Source: CAD feature listing. Evaluate the final solid. Frame: model axes, mm. A direction names the side the tool comes from. Give positions to 0.01 mm unless a question says otherwise; leave off trailing zeros. Loops run counter-clockwise (first coordinate to the right, second up) from the corner with the lowest first, then second, coordinate; pieces in that order, holes last. Notation, with made-up numbers: (-20, 81) - (13, 81) arc R23 cw to (13, 112) - close; hole circle Ø7 at (23.25, 8). An arc over 180 degrees is marked (long way). Put each result on its own line as item: value.
```python
from build123d import *

# Parameters (mm, degrees)
SKETCH1_W            = 152.4
SKETCH1_H            = 254
BOSS_EXTRUDE1_DEPTH  = 12.7
SKETCH2_W            = 38.1
SKETCH2_H            = 19.05
CUT_EXTRUDE1_DEPTH   = 149.649688866
FILLET1_R            = 3.302
FILLET1_OF_MIRROR1_R = 3.302
FILLET2_R            = 3.302


with BuildPart() as part:
    # Sketch1 → Boss-Extrude1 (new body)
    with BuildSketch(Plane(origin=(0, 0, 0), x_dir=(1, 0, 0), z_dir=(0, 1, 0))):
        Rectangle(SKETCH1_W, SKETCH1_H)
    extrude(amount=BOSS_EXTRUDE1_DEPTH)

    # Sketch2 → Cut-Extrude1 (cut, through all)
    with BuildSketch(Plane(origin=(0, 12.7, 0), x_dir=(1, 0, 0), z_dir=(0, 1, 0))):
        with Locations((57.15, -66.675)):
            Rectangle(SKETCH2_W, SKETCH2_H)
    cut_extrude1 = extrude(amount=-CUT_EXTRUDE1_DEPTH, mode=Mode.SUBTRACT)

    # Fillet1
    fillet1_edges = [part.edges().sort_by_distance(p)[0] for p in [
        (38.1, 6.35, 76.2),
        (38.1, 6.35, 57.15),
    ]]
    fillet(fillet1_edges, radius=FILLET1_R)

    # Mirror1: Cut-Extrude1 across plane
    add(cut_extrude1.mirror(Plane(origin=(0, 0, 0), x_dir=(0, 0, 1), z_dir=(1, 0, 0))), mode=Mode.SUBTRACT)

    # Fillet1 of Mirror1
    fillet1_of_mirror1_edges = [part.edges().sort_by_distance(p)[0] for p in [
        (-38.1, 6.35, 76.2),
        (-38.1, 6.35, 57.15),
    ]]
    fillet(fillet1_of_mirror1_edges, radius=FILLET1_OF_MIRROR1_R)

    # Fillet2
    fillet2_edges = [part.edges().sort_by_distance(p)[0] for p in [
        (76.2, 6.35, 57.15),
        (76.2, 6.35, 76.2),
        (-76.2, 6.35, 76.2),
        (-76.2, 6.35, 57.15),
        (76.2, 6.35, 127),
        (-76.2, 6.35, 127),
        (-76.2, 6.35, -127),
        (76.2, 6.35, -127),
    ]]
    fillet(fillet2_edges, radius=FILLET2_R)


solid = part.part
```
1) Section query A-A, the plane x = 58. Output: boundary loops of the cut face in (y, z), plus the area to 3 significant figures.
Check result:
outline: (0, -127) - (12.7, -127) - (12.7, 57.15) - (0, 57.15) - close; (0, 76.2) - (12.7, 76.2) - (12.7, 127) - (0, 127) - close
area: 2,980 mm²
2) Pin query (flat end, axial travel): P1, Ø6, axis at y = 8.5, z = 68.5, coming from the +X side. Return the tip coordinate at first contact, or that it passes through.
Check result:
P1: x = 38.1
3) Section query B-B, the plane y = 5.75. Output: boundary loops of the cut face in (x, z), plus the area to 3 significant figures.
Check result:
outline: (-76.2, -123.7) arc R3.3 ccw to (-72.9, -127) - (72.9, -127) arc R3.3 ccw to (76.2, -123.7) - (76.2, 53.85) arc R3.3 ccw to (72.9, 57.15) - (41.4, 57.15) arc R3.3 cw to (38.1, 60.45) - (38.1, 72.9) arc R3.3 cw to (41.4, 76.2) - (72.9, 76.2) arc R3.3 ccw to (76.2, 79.5) - (76.2, 123.7) arc R3.3 ccw to (72.9, 127) - (-72.9, 127) arc R3.3 ccw to (-76.2, 123.7) - (-76.2, 79.5) arc R3.3 ccw to (-72.9, 76.2) - (-41.4, 76.2) arc R3.3 cw to (-38.1, 72.9) - (-38.1, 60.45) arc R3.3 cw to (-41.4, 57.15) - (-72.9, 57.15) arc R3.3 ccw to (-76.2, 53.85) - close
area: 37,200 mm²
4) Material intervals for line 1 along Z through (x, y) = (-65.5, 8.75); line 2 along X through (y, z) = (6.5, 65), sorted ascending. Write a range as [from, to].
Check result:
line 1: [-127, 57.15], [76.2, 127]
line 2: [-38.1, 38.1]
5) Access query for faces 1 (the flat face through (-38.1, 6, 67)), 2 (the flat face through (38.1, 6, 67)), 3 (the flat face through (76.2, 6, 102)). Directions: +Z, -Z, +X, -X, +Y, -Y. A direction counts if a zero-diameter tool reaches every point of the face in a straight line with its end or side. Return the directions, or none.
Check result:
face 1: -X, +Y, -Y
face 2: +X, +Y, -Y
face 3: +Z, -Z, +X, +Y, -Y
